The drawing under review shows one solid part. Ordinate dimensions are in mm from its lowest x, y, z. A direction names the side the tool comes from. Round coordinates to 2 decimals unless told otherwise and drop trailing zeros. Write each loop counter-clockwise with the first axis right and the second up, starting at its lowest first coordinate (ties: lowest second). Pieces come first, ordered by that corner, then holes. Notation, with made-up numbers: (-10, 69.25) -> (-5, 69.25) arc R21 ccw to (-5, 100.25) -> close; hole circle Ø7 at (37, 36.5). An arc over 180 degrees is marked (long way). Use CSV: the item, a comma, the result in double quotes. Start each with the question number.
1) Take a section at C-C, the plane z = 21.25. Give the boundary of the cut face in (x, y), then the cut area to 3 significant figures.
2) Wall thickness on probe 1 along Z at (x, y) = (1.5, 19.5); probe 2 along Y at (x, z) = (15, 15.5); probe 3 along Z at (x, y) = (25.5, 9): over which ranges is each line inside the solid? List them lowest first. Write a range as [from, to].
3) Take a section at D-D, the plane y = 25.5. Give the boundary of the cut face in (x, z).
4) For pin 1 Ø2 at (x, z) = (16, 22.5) entering from +Y; pin 2 Ø1 at (x, y) = (9, 23.5) entering from +Z; pin 3 Ø10 at (y, z) = (17.5, 22) entering from +X, all flat-tipped, find the tip position at first contact; note any pin that passes through.
5) Take a section at B-B, the plane y = 21.5. Give the boundary of the cut face in (x, z) (1 decimal), then the cut area to 3 significant figures.
6) Take a section at A-A, the plane x = 15. Give the boundary of the cut face in (y, z) (3 decimals).
7) Machinability: for the marked faces 1 and 2, which of the approach directions +Z, -Z, +X, -X, +Y, -Y give a long, thin tool a straight path to every point of the face, cutting with its end or side? Answer none if there is none.
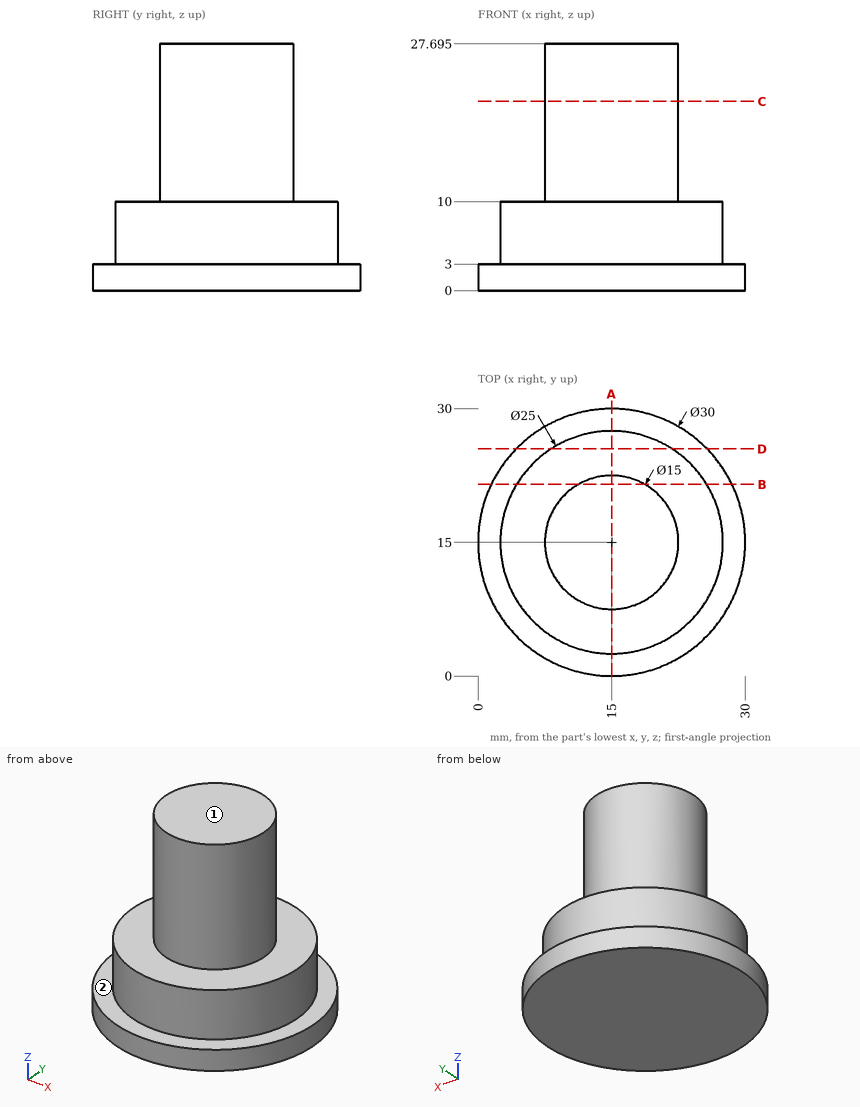
Values found:
1,outline,"circle Ø15 at (15, 15)"
1,area,"177 mm²"
2,probe 1,"[0, 3]"
2,probe 2,"[7.5, 22.5]"
2,probe 3,"[0, 10]"
3,outline,"(4.29, 0) -> (25.71, 0) -> (25.71, 3) -> (21.78, 3) -> (21.78, 10) -> (8.22, 10) -> (8.22, 3) -> (4.29, 3) -> close"
4,pin 1,"y = 22.5"
4,pin 2,"z = 10"
4,pin 3,"x = 22.5"
5,outline,"(1.5, 0) -> (28.5, 0) -> (28.5, 3) -> (25.7, 3) -> (25.7, 10) -> (18.7, 10) -> (18.7, 27.7) -> (11.3, 27.7) -> (11.3, 10) -> (4.3, 10) -> (4.3, 3) -> (1.5, 3) -> close"
5,area,"363 mm²"
6,outline,"(0, 0) -> (30, 0) -> (30, 3) -> (27.5, 3) -> (27.5, 10) -> (22.5, 10) -> (22.5, 27.695) -> (7.5, 27.695) -> (7.5, 10) -> (2.5, 10) -> (2.5, 3) -> (0, 3) -> close"
7,face 1,"+Z, +X, -X, +Y, -Y"
7,face 2,"+Z"
